For this review, take the finished solid that the model builds, in its own axes (mm). Coordinates: 2 decimals unless noted, no trailing zeros. Loops run counter-clockwise (first coordinate to the right, second up) from the corner with the lowest first, then second, coordinate; pieces in that order, holes last. Notation, with made-up numbers: M 46.5,-21 L 61.5,-21 A8 cw 61.5,-16 Z; hole C 7.5,29 d9. An arc over 180 degrees is marked long. Put each result on its own line as item: value.
```python
from build123d import *

# Parameters (mm, degrees)
SKETCH_1_W          = 110
SKETCH_1_H          = 150
EXTRUDE_1_DEPTH     = 3
SKETCH_2_R          = 1.5
CUT_EXTRUDE_1_DEPTH = 3
SKETCH_3_R          = 2
CUT_EXTRUDE_2_DEPTH = 187.034942954
SKETCH_4_R          = 1.5
CUT_EXTRUDE_3_DEPTH = 187.034942954
CUT_EXTRUDE_4_DEPTH = 10


with BuildPart() as part:
    # 草图1 → 凸台-拉伸1 (new body)
    with BuildSketch(Plane.XY):
        with Locations((55, 75)):
            Rectangle(SKETCH_1_W, SKETCH_1_H)
    extrude(amount=EXTRUDE_1_DEPTH)

    # 草图2 → 切除-拉伸1 (cut)
    with BuildSketch(Plane.XY.offset(3)):
        with Locations((45, 147)):
            Circle(SKETCH_2_R)
        with Locations((25, 147)):
            Circle(SKETCH_2_R)
        with Locations(Location((85, 147, 0), (0, 0, 180))):
            Circle(SKETCH_2_R)
        with Locations(Location((65, 147, 0), (0, 0, 180))):
            Circle(SKETCH_2_R)
    extrude(amount=-CUT_EXTRUDE_1_DEPTH, mode=Mode.SUBTRACT)

    # 草图3 → 切除-拉伸2 (cut, through all)
    with BuildSketch(Plane.XY.offset(3)):
        with Locations((3.8, 47)):
            Circle(SKETCH_3_R)
        with Locations((3.8, 30)):
            Circle(SKETCH_3_R)
        with Locations(Location((106.2, 30, 0), (0, 0, 180))):
            Circle(SKETCH_3_R)
        with Locations(Location((106.2, 47, 0), (0, 0, 180))):
            Circle(SKETCH_3_R)
        with Locations((106.2, 103)):
            Circle(SKETCH_3_R)
        with Locations((106.2, 120)):
            Circle(SKETCH_3_R)
        with Locations(Location((3.8, 120, 0), (0, 0, 180))):
            Circle(SKETCH_3_R)
        with Locations(Location((3.8, 103, 0), (0, 0, 180))):
            Circle(SKETCH_3_R)
    extrude(amount=-CUT_EXTRUDE_2_DEPTH, mode=Mode.SUBTRACT)

    # 草图4 → 切除-拉伸3 (cut, through all)
    with BuildSketch(Plane.XY.offset(3)):
        with Locations((63, 3)):
            Circle(SKETCH_4_R)
        with Locations((83, 3)):
            Circle(SKETCH_4_R)
        with Locations(Location((27, 3, 0), (0, 0, 180))):
            Circle(SKETCH_4_R)
        with Locations(Location((47, 3, 0), (0, 0, 180))):
            Circle(SKETCH_4_R)
    extrude(amount=-CUT_EXTRUDE_3_DEPTH, mode=Mode.SUBTRACT)

    # 草图5 → 切除-拉伸4 (cut)
    with BuildSketch(Plane.XY.offset(3)):
        with BuildLine():
            Line((22.319382164, 135.252792574), (44.525443001, 135.252792574))
            ThreePointArc((44.525443001, 135.252792574), (50.525443001, 129.252792574), (44.525443001, 123.252792574))
            Line((44.525443001, 123.252792574), (22.319382164, 123.252792574))
            ThreePointArc((22.319382164, 123.252792574), (16.319382164, 129.252792574), (22.319382164, 135.252792574))
        make_face()
        with BuildLine():
            Line((22.319382164, 110.252792574), (44.525443001, 110.252792574))
            ThreePointArc((44.525443001, 110.252792574), (50.525443001, 104.252792574), (44.525443001, 98.252792574))
            Line((44.525443001, 98.252792574), (22.319382164, 98.252792574))
            ThreePointArc((22.319382164, 98.252792574), (16.319382164, 104.252792574), (22.319382164, 110.252792574))
        make_face()
        with BuildLine():
            Line((22.319382164, 85.252792574), (44.525443001, 85.252792574))
            ThreePointArc((44.525443001, 85.252792574), (50.525443001, 79.252792574), (44.525443001, 73.252792574))
            Line((44.525443001, 73.252792574), (22.319382164, 73.252792574))
            ThreePointArc((22.319382164, 73.252792574), (16.319382164, 79.252792574), (22.319382164, 85.252792574))
        make_face()
        with BuildLine():
            Line((22.319382164, 60.252792574), (44.525443001, 60.252792574))
            ThreePointArc((44.525443001, 60.252792574), (50.525443001, 54.252792574), (44.525443001, 48.252792574))
            Line((44.525443001, 48.252792574), (22.319382164, 48.252792574))
            ThreePointArc((22.319382164, 48.252792574), (16.319382164, 54.252792574), (22.319382164, 60.252792574))
        make_face()
        with BuildLine():
            Line((22.319382164, 35.252792574), (44.525443001, 35.252792574))
            ThreePointArc((44.525443001, 35.252792574), (50.525443001, 29.252792574), (44.525443001, 23.252792574))
            Line((44.525443001, 23.252792574), (22.319382164, 23.252792574))
            ThreePointArc((22.319382164, 23.252792574), (16.319382164, 29.252792574), (22.319382164, 35.252792574))
        make_face()
        with BuildLine():
            Line((87.680617836, 35.252792574), (65.474556999, 35.252792574))
            ThreePointArc((65.474556999, 35.252792574), (59.474556999, 29.252792574), (65.474556999, 23.252792574))
            Line((65.474556999, 23.252792574), (87.680617836, 23.252792574))
            ThreePointArc((87.680617836, 23.252792574), (93.680617836, 29.252792574), (87.680617836, 35.252792574))
        make_face()
        with BuildLine():
            Line((87.680617836, 60.252792574), (65.474556999, 60.252792574))
            ThreePointArc((65.474556999, 60.252792574), (59.474556999, 54.252792574), (65.474556999, 48.252792574))
            Line((65.474556999, 48.252792574), (87.680617836, 48.252792574))
            ThreePointArc((87.680617836, 48.252792574), (93.680617836, 54.252792574), (87.680617836, 60.252792574))
        make_face()
        with BuildLine():
            Line((87.680617836, 85.252792574), (65.474556999, 85.252792574))
            ThreePointArc((65.474556999, 85.252792574), (59.474556999, 79.252792574), (65.474556999, 73.252792574))
            Line((65.474556999, 73.252792574), (87.680617836, 73.252792574))
            ThreePointArc((87.680617836, 73.252792574), (93.680617836, 79.252792574), (87.680617836, 85.252792574))
        make_face()
        with BuildLine():
            Line((87.680617836, 110.252792574), (65.474556999, 110.252792574))
            ThreePointArc((65.474556999, 110.252792574), (59.474556999, 104.252792574), (65.474556999, 98.252792574))
            Line((65.474556999, 98.252792574), (87.680617836, 98.252792574))
            ThreePointArc((87.680617836, 98.252792574), (93.680617836, 104.252792574), (87.680617836, 110.252792574))
        make_face()
        with BuildLine():
            Line((87.680617836, 135.252792574), (65.474556999, 135.252792574))
            ThreePointArc((65.474556999, 135.252792574), (59.474556999, 129.252792574), (65.474556999, 123.252792574))
            Line((65.474556999, 123.252792574), (87.680617836, 123.252792574))
            ThreePointArc((87.680617836, 123.252792574), (93.680617836, 129.252792574), (87.680617836, 135.252792574))
        make_face()
    extrude(amount=-CUT_EXTRUDE_4_DEPTH, mode=Mode.SUBTRACT)


solid = part.part
```
(1) Add section C-C (y = 30). Write out the cut boundary in (x, z).
Determined:
outline: M 0,0 L 1.8,0 L 1.8,3 L 0,3 Z; M 5.8,0 L 16.37,0 L 16.37,3 L 5.8,3 Z; M 50.48,0 L 59.52,0 L 59.52,3 L 50.48,3 Z; M 93.63,0 L 104.2,0 L 104.2,3 L 93.63,3 Z; M 108.2,0 L 110,0 L 110,3 L 108.2,3 Z
(2) For pin 1 (3.5 mm diameter, centred on x = 106.2, y = 120, fed in from +Z), flat-tipped, find the tip position at first contact; note if it passes through.
Determined:
pin 1: passes through
(3) Draft analysis for pull direction Y (two halves, no side actions). For faces 1 (the flat face through (0, 74, 1)), 2 (the flat face through (76, 73.253, 2)), state which applies: +Y half, -Y half, draft (parallel to the pull), parting line (faces both ways), or undercut.
Determined:
face 1: draft
face 2: undercut
(4) Add section D-D (z = 0.7). State how many separate pieces and enclosed holes the cut face has, plus the area to 3 significant figures.
Determined:
separate pieces: 1
enclosed holes: 26
area: 12,500 mm^2
(5) Wall thickness on line 1 along Y through (x, z) = (3.8, 1.4); line 2 along X through (y, z) = (147, 1.5); line 3 along X through (y, z) = (80.5, 0.4): over which ranges is each line inside the solid? List them lowest first. Write a range as [from, to].
Determined:
line 1: y = [0, 28], [32, 45], [49, 101], [105, 118], [122, 150]
line 2: x = [0, 23.5], [26.5, 43.5], [46.5, 63.5], [66.5, 83.5], [86.5, 110]
line 3: x = [0, 16.45], [50.39, 59.61], [93.55, 110]
(6) Add section B-B (y = 120). Write out the cut boundary in (x, z), plus the area to 3 significant figures.
Determined:
outline: M 0,0 L 1.8,0 L 1.8,3 L 0,3 Z; M 5.8,0 L 104.2,0 L 104.2,3 L 5.8,3 Z; M 108.2,0 L 110,0 L 110,3 L 108.2,3 Z
area: 306 mm^2
(7) Add section A-A (x = 42). Write out the cut boundary in (y, z).
Determined:
outline: M 0,0 L 23.25,0 L 23.25,3 L 0,3 Z; M 35.25,0 L 48.25,0 L 48.25,3 L 35.25,3 Z; M 60.25,0 L 73.25,0 L 73.25,3 L 60.25,3 Z; M 85.25,0 L 98.25,0 L 98.25,3 L 85.25,3 Z; M 110.25,0 L 123.25,0 L 123.25,3 L 110.25,3 Z; M 135.25,0 L 150,0 L 150,3 L 135.25,3 Z
